from build123d import *

# Parameters (mm, degrees)
TAP_DRILL_FOR_M3_TAP1_D     = 2.5
TAP_DRILL_FOR_M3_TAP1_DEPTH = 5.5
TAP_DRILL_FOR_M3_TAP1_TIP   = 0.751075774


with BuildPart() as part:
    # Sketch2 → Revolve4 (revolve)
    with BuildSketch(Plane.XY):
        Polygon((296.055680528, 81.106851928), (303.855680528, 81.106851928), (304.055680528, 81.406851928), (312.055680528, 81.406851928), (312.055680528, 79.406851928), (312.055680528, 76.706851928), (277.446915198, 76.706851928), (277.446915198, 78.436851928), (294.046915198, 78.436851928), (309.446915198, 78.436851928), (309.446915198, 81.106851928), (304.216235656, 81.106851928), (304.016235656, 80.806851928), (296.100980113, 80.806851928), (294.055680528, 80.174765167), (294.055680528, 80.488764715), align=None)
    revolve(axis=Axis((277.446915198, 76.706851928, 0), (1, 0, 0)))

    # Tap Drill for M3 Tap1
    with Locations(Plane(origin=(312.055680528, 0, 0), x_dir=(0, 0, -1), z_dir=(1, 0, 0))):
        with Locations((0, 76.706851928)):
            Hole(TAP_DRILL_FOR_M3_TAP1_D / 2, depth=TAP_DRILL_FOR_M3_TAP1_DEPTH)
            with Locations((0, 0, -(TAP_DRILL_FOR_M3_TAP1_DEPTH + TAP_DRILL_FOR_M3_TAP1_TIP / 2))):  # 118° drill point
                Cone(0, TAP_DRILL_FOR_M3_TAP1_D / 2, TAP_DRILL_FOR_M3_TAP1_TIP, mode=Mode.SUBTRACT)


solid = part.part
Part model, mm, in its own coordinate system. A direction names the side the tool comes from. Round coordinates to 2 decimals unless told otherwise and drop trailing zeros. Order: outer loops, then holes, each group sorted by start corner. A loop starts at its lowest first (then second) coordinate and runs counter-clockwise, first axis right, second up. Notation, with made-up numbers: (-11.75, 45.5) -> (1.25, 45.5) arc R13 ccw to (1.25, 69.5) -> close; hole circle Ø4 at (38, 35.25). An arc over 180 degrees is marked (long way). Put each result on its own line as item: value.
Q1. Pull direction X, two halves, no side cores. Call faces 1 (the face through (300.01, 72.31, 0.19)), 2 (the face through (277.447, 77, 0)), 3 (the face through (306.79, 72.31, 0.19)), 4 (the face through (309.447, 74.8, 0.1)): pulls with the +X half, pulls with the -X half, needs draft (parallel to the pull), parting line crosses it, or undercut.
From the geometry:
face 1: needs draft
face 2: pulls with the -X half
face 3: undercut
face 4: undercut
Q2. Pin check, flat tips, straight feed: pin 1 Ø1 at (x, y) = (304.5, 75) entering from -Z; pin 2 Ø3 at (x, y) = (291, 74.5) entering from +Z; pin 3 Ø1.5 at (x, y) = (295, 80) entering from +Z. Stop position of each tip, or through.
From the geometry:
pin 1: stops at z = -4.54
pin 2: stops at z = 1.58
pin 3: stops at z = 3.25
Q3. Band-saw the part on A-A (x = 305.5). Give the cut face in (y, z).
From the geometry:
outline: circle Ø9.4 at (76.71, 0); circle Ø3.46 at (76.71, 0); hole circle Ø8.8 at (76.71, 0)
Q4. Band-saw the part on B-B (x = 283.5). Give the cut face in (y, z), and give its area (3 significant figures).
From the geometry:
outline: circle Ø3.46 at (76.71, 0)
area: 9.40 mm2
Q5. Tool access for faces 5 (the face through (300.003, 80.494, -1.57)), 6 (the face through (312.056, 75.7, -1)), 7 (the face through (293.223, 78.305, -0.663)), 8 (the face through (308.11, 81.19, 1.41)), 9 (the face through (309.27, 75.6, 0.58)): list every direction of +Z, -Z, +X, -X, +Y, -Y with a clear straight run to the whole face (end or side of a thin tool).
From the geometry:
face 5: none
face 6: +Z, -Z, +X, +Y, -Y
face 7: -X
face 8: +X, -X
face 9: +X
Q6. Band-saw the part on C-C (x = 299). Give the cut face in (y, z).
From the geometry:
outline: circle Ø8.8 at (76.71, 0); circle Ø3.46 at (76.71, 0); hole circle Ø8.2 at (76.71, 0)
Q7. Wall check: line 1 (Y direction, x = 303, z = -0.5); line 2 (X direction, y = 76.5, z = 3); line 3 (Y direction, x = 303.5, z = -3.5). Give the ranges that are in metal, low to high. Write a range as [from, to].
From the geometry:
line 1: y = [72.34, 72.64], [75.05, 78.36], [80.78, 81.08]
line 2: x = [309.45, 312.06]
line 3: y = [74.04, 74.57], [78.84, 79.37]
